```python
from build123d import *

# Parameters (mm, degrees)
PAD_DEPTH       = 30
SKETCH001_W     = 14.2
SKETCH001_H     = 24
POCKET_DEPTH    = 19
SKETCH002_R     = 3.15
POCKET001_DEPTH = 5
SKETCH003_W     = 14.2
SKETCH003_H     = 5
POCKET002_DEPTH = 5
SKETCH004_W     = 20
SKETCH004_H     = 10
SKETCH004_W_2   = 14.2
SKETCH004_H_2   = 5
PAD001_DEPTH    = 15
PAD001_TAPER    = 3
SKETCH005_R     = 3.5
POCKET003_DEPTH = 15


with BuildPart() as part:
    # Sketch → Pad (new body)
    with BuildSketch(Plane.XY):
        with BuildLine():
            ThreePointArc((-7.1, 0), (-12.1, 5), (-17.1, 0))
            ThreePointArc((-17.1, 0), (-15.221859, -7.791341), (-10, -13.871193))
            Line((-10, -13.871193), (-10, -21.871193))
            Line((-10, -21.871193), (10, -21.871193))
            Line((10, -13.871193), (10, -21.871193))
            ThreePointArc((10, -13.871193), (15.221859, -7.791341), (17.1, 0))
            ThreePointArc((17.1, 0), (12.1, 5), (7.1, 0))
            ThreePointArc((-7.1, 0), (0, -7.1), (7.1, 0))
        make_face()
        Polygon((-9.5, -1.501111), (-9.5, 1.501111), (-12.1, 3.002221), (-14.7, 1.501111), (-14.7, -1.501111), (-12.1, -3.002221), align=None, mode=Mode.SUBTRACT)
        Polygon((14.7, -1.501111), (14.7, 1.501111), (12.1, 3.002221), (9.5, 1.501111), (9.5, -1.501111), (12.1, -3.002221), align=None, mode=Mode.SUBTRACT)
    extrude(amount=PAD_DEPTH)

    # Sketch001 (on DatumPlane) → Pocket (cut)
    with BuildSketch(Plane.XZ.offset(-0.128807)):
        with Locations((0, 15)):
            Rectangle(SKETCH001_W, SKETCH001_H)
    extrude(amount=POCKET_DEPTH, mode=Mode.SUBTRACT)

    # Sketch002 (on Face13 of Pocket) → Pocket001 (cut)
    with BuildSketch(Plane.XZ.offset(21.871193)):
        with Locations((0, 7.5)):
            Circle(SKETCH002_R)
    extrude(amount=-POCKET001_DEPTH, mode=Mode.SUBTRACT)

    # Sketch003 (on Face10 of Pocket001) → Pocket002 (cut)
    with BuildSketch(Plane(origin=(0, -18.871193, 0), x_dir=(-1, 0, 0), z_dir=(0, 1, 0))):
        with Locations((0, 19)):
            Rectangle(SKETCH003_W, SKETCH003_H)
    extrude(amount=-POCKET002_DEPTH, mode=Mode.SUBTRACT)

    # Sketch004 (on Face15 of Pocket002) → Pad001 (join)
    with BuildSketch(Plane.XZ.offset(21.871193)):
        with Locations((0, 19.5)):
            Rectangle(SKETCH004_W, SKETCH004_H)
        with Locations((0, 19)):
            Rectangle(SKETCH004_W_2, SKETCH004_H_2, mode=Mode.SUBTRACT)
    extrude(amount=PAD001_DEPTH, taper=PAD001_TAPER)

    # Sketch005 (on Face7 of Pad001) → Pocket003 (cut)
    with BuildSketch(Plane.XY.offset(30)):
        with Locations((-12.1, 0)):
            Circle(SKETCH005_R)
        with Locations((12.1, 0)):
            Circle(SKETCH005_R)
    extrude(amount=-POCKET003_DEPTH, mode=Mode.SUBTRACT)


solid = part.part
```
Here's how the part is built. I have some questions about the finished solid (model axes, mm). A direction names the side the tool comes from. Round coordinates to 2 decimals unless told otherwise and drop trailing zeros. Write each loop counter-clockwise with the first axis right and the second up, starting at its lowest first coordinate (ties: lowest second). Pieces come first, ordered by that corner, then holes.
Q1. Which directions (+Z, -Z, +X, -X, +Y, -Y) give clear straight access to the entire face, cutting with the end or side of a thin tool? Please do faces 5 (the flat face through (0, -11, 3)), 6 (the flat face through (0, -20, 21.5)), 7 (the flat face through (-10.818, -2.262, 7.395)).
Q2. If we section it at C-C on x = -11: Write out the boundary of the cut face in (y, z), plus the area to 3 significant figures.
Q3. Will these pins go through, and if not, where does the flat tip stop? P1, Ø12, axis at x = 11.5, y = -29.5, coming from the -Z side; P2, Ø8, axis at x = 0, z = 7.5, coming from the -Y side; P3, Ø9, axis at y = -18.5, z = 19, coming from the -X side.
Q4. If we section it at D-D on y = -4: Write out the boundary of the cut face in (x, z), plus the area to 3 significant figures.
Q5. If we section it at A-A on y = -21: Write out the boundary of the cut face in (x, z).
Q6. Please list where these lines run through material, in increasing order: probe 1 along Z at (x, y) = (0, -19.6); probe 2 along X at (y, z) = (-7, 9.5); probe 3 along X at (y, z) = (-15, 4).
Q7. If we mould it in two halves opening along Z, with no side actions, what happens to faces 1 (the flat face through (0, -8, 0)), 2 (the cylindrical face through (-12, 5, 15)), 3 (the flat face through (0, -8, 30)), 4 (the flat face through (0, -18.871, 24))? For each: +Z half, -Z half, draft (parallel to the pull), parting line (faces both ways), or undercut.
Q8. If we section it at B-B on z = 7.5: Write out the boundary of the cut face in (x, y).
Answer below:
1. face 5: +Y
1. face 6: +Y, -Y
1. face 7: +Z, -Z
2. outline: (-13.09, 0) - (-2.37, 0) - (-2.37, 15) - (-3.32, 15) - (-3.32, 30) - (-13.09, 30) - close; (2.37, 0) - (4.88, 0) - (4.88, 30) - (3.32, 30) - (3.32, 15) - (2.37, 15) - close
2. area: 368 mm2
3. P1: stops at z = 14.6
3. P2: stops at y = -21.87
3. P3: stops at x = -10
4. outline: (-16.63, 0) - (-5.87, 0) - (-5.87, 3) - (-7.1, 3) - (-7.1, 27) - (-5.87, 27) - (-5.87, 30) - (-16.63, 30) - close; (5.87, 0) - (16.63, 0) - (16.63, 30) - (5.87, 30) - (5.87, 27) - (7.1, 27) - (7.1, 3) - (5.87, 3) - close
4. area: 586 mm2
5. outline: (-10, 0) - (10, 0) - (10, 30) - (-10, 30) - close; hole (-7.1, 16.5) - (7.1, 16.5) - (7.1, 21.5) - (-7.1, 21.5) - close; hole circle Ø6.3 at (0, 7.5)
6. probe 1: z = 0 to 4.35, 10.65 to 16.5, 21.5 to 30
6. probe 2: x = -15.6 to -7.1, 7.1 to 15.6
6. probe 3: x = -10 to -7.1, 7.1 to 10
7. face 1: -Z half
7. face 2: draft
7. face 3: +Z half
7. face 4: undercut
8. outline: (-17.1, 0) arc R17.1 ccw to (-10, -13.87) - (-10, -21.87) - (-3.15, -21.87) - (-3.15, -18.87) - (-7.1, -18.87) - (-7.1, 0) arc R5 ccw to start; (3.15, -21.87) - (10, -21.87) - (10, -13.87) arc R17.1 ccw to (17.1, 0) arc R5 ccw to (7.1, 0) - (7.1, -18.87) - (3.15, -18.87) - close; hole (-14.7, -1.5) - (-12.1, -3) - (-9.5, -1.5) - (-9.5, 1.5) - (-12.1, 3) - (-14.7, 1.5) - close; hole (9.5, -1.5) - (12.1, -3) - (14.7, -1.5) - (14.7, 1.5) - (12.1, 3) - (9.5, 1.5) - close
